Source: CAD feature listing. Evaluate the final solid. Frame: model axes, mm. Give positions to 0.01 mm unless a question says otherwise; leave off trailing zeros. Loops run counter-clockwise (first coordinate to the right, second up) from the corner with the lowest first, then second, coordinate; pieces in that order, holes last. Notation, with made-up numbers: (10.5, 57.5) -> (15.5, 57.5) arc R31 ccw to (15.5, 94.5) -> close; hole circle Ø11 at (58.25, 47). An arc over 180 degrees is marked (long way). Return JSON: item names as keys, results as strings. Group by question number.
(1) Cut plane C-C on x = -1.3. Return loops of the section in (y, z), then the cut area to 3 significant figures.
(2) Pin query (flat end, axial travel): pin 1 (1 mm diameter, centred on x = -1, y = -0.5, fed in from +Z). Return the tip coordinate at first contact, or that it passes through.
(3) Ray query, line 1 (Z direction, x = -0.9, y = 2.75); line 2 (Z direction, x = -0.9, y = 4.5); line 3 (Y direction, x = -1.9, z = 12.25). Return the intervals inside material, ascending. Write a range as from..to.
(4) Cut plane A-A on y = 2.75. Return loops of the section in (x, z).
(5) Cut plane D-D on z = 3.75. Return loops of the section in (x, y), then the cut area to 3 significant figures.
(6) Cut plane B-B on z = 12.5. Return loops of the section in (x, y).
(7) Draft query along Y for faces 1 (the face through (-1.014, 2.392, 12.727)), 2 (the face through (0, 2, 6)), 3 (the face through (-1.01, 1.3, 14.26)). Return one class per face: released by +Y, released by -Y, zero draft, split by the parting line, or undercut.
```python
from build123d import *

# Parameters (mm, degrees)
SKETCH106_R      = 2.75
EXTRUDE024_DEPTH = 5
EXTRUDE023_DEPTH = 15
EXTRUDE022_DEPTH = 2


with BuildPart() as extrude024:
    # Sketch106 → Extrude024 (new body)
    with BuildSketch(Plane.YZ.offset(-2)):
        with Locations((2.75, 10)):
            Circle(SKETCH106_R)
    extrude(amount=EXTRUDE024_DEPTH)


with BuildPart() as extrude023:
    # Sketch105 → Extrude023 (new body)
    with BuildSketch(Plane.XY):
        Polygon((0, 5.5), (-1.75, 7.25), (0, 7.25), align=None)
    extrude(amount=EXTRUDE023_DEPTH)


with BuildPart() as cut019:
    # Sketch104 → Extrude022 (new body)
    with BuildSketch(Plane.YZ.offset(-2)):
        with BuildLine():
            Line((-1.75, 0), (7.25, 0))
            Line((7.25, 0), (7.25, 10))
            ThreePointArc((7.25, 10), (2.749999, 14.5), (-1.75, 9.999998))
            Line((-1.75, 0), (-1.75, 9.999998))
        make_face()
    extrude(amount=EXTRUDE022_DEPTH)

    # Cut018: cut Extrude023
    add(extrude023.part, mode=Mode.SUBTRACT)

    # Cut019: cut Extrude024
    add(extrude024.part, mode=Mode.SUBTRACT)


solid = cut019.part
```
Answers:
{
 "1": {"outline": "(-1.75, 0) -> (6.8, 0) -> (6.8, 11.96) arc R4.5 ccw to (-1.75, 10) -> close; hole circle Ø5.5 at (2.75, 10)", "area": "93.0 mm²"},
 "2": {"pin 1": "z = 13.56"},
 "3": {"line 1": "0..7.25, 12.75..14.5", "line 2": "0..7.88, 12.12..14.15", "line 3": "-1.15..1.17, 4.33..6.65"},
 "4": {"outline": "(-2, 0) -> (0, 0) -> (0, 7.25) -> (-2, 7.25) -> close; (-2, 12.75) -> (0, 12.75) -> (0, 14.5) -> (-2, 14.5) -> close"},
 "5": {"outline": "(-2, -1.75) -> (0, -1.75) -> (0, 5.5) -> (-1.75, 7.25) -> (-2, 7.25) -> close", "area": "16.5 mm²"},
 "6": {"outline": "(-2, -0.99) -> (0, -0.99) -> (0, 1.6) -> (-2, 1.6) -> close; (-2, 3.9) -> (0, 3.9) -> (0, 5.5) -> (-0.99, 6.49) -> (-2, 6.49) -> close"},
 "7": {"face 1": "undercut", "face 2": "zero draft", "face 3": "split by the parting line"}
}
